from build123d import *

# Parameters (mm, degrees)
F0_R     = 9
F0_R_2   = 4
F1_DEPTH = 1.5
F2_DEPTH = 4
F3_R     = 2.35
F4_DEPTH = 2.5


# Not quite as in the source:
# - a feature names something its author has since deleted; it is built from what else it names


with BuildPart() as f1:
    # F0 (on Top) → F1 (new body)
    with BuildSketch(Plane.XY):
        Circle(F0_R)
        Circle(F0_R_2, mode=Mode.SUBTRACT)
        Circle(F0_R_2)
    extrude(amount=-F1_DEPTH)

    # F0 (on Top) → F2 (join)
    with BuildSketch(Plane.XY):
        Circle(F0_R_2)
    extrude(amount=F2_DEPTH)

    # F3 (on face) → F4 (join)
    with BuildSketch(Plane.XY.offset(4)):
        Circle(F3_R)
    extrude(amount=F4_DEPTH)


solid = f1.part
Read the model definition and answer for the solid it produces. Units are mm, in the model's axes. A direction names the side the tool comes from. Give positions to 0.01 mm unless a question says otherwise; leave off trailing zeros. Write each loop counter-clockwise with the first axis right and the second up, starting at its lowest first coordinate (ties: lowest second). Pieces come first, ordered by that corner, then holes. Notation, with made-up numbers: (-6.75, 66.25) - (49.25, 66.25) arc R13 ccw to (49.25, 85.25) - close; hole circle Ø4 at (81.25, 57). An arc over 180 degrees is marked (long way). Use CSV: the item, a comma, the result in double quotes. Start each with the question number.
(1) Consider line 1 along Z through (x, y) = (4.5, -6); line 2 along Y through (x, z) = (-0.25, 4.25); line 3 along Y through (x, z) = (0.5, 1.75). Determine where each line is inside the solid, lowest interval first.
(2) For faces 1 (the cylindrical face through (-1.172, 8.923, -0.74)), 2 (the cylindrical face through (-0.509, -2.294, 5.232)), determine the directions among +Z, -Z, +X, -X, +Y, -Y from which every point of the face is accessible in a straight line to the end or side of a thin tool.
(3) Given P1, Ø4, axis at x = 1.5, z = 2.5, coming from the +Y side; P2, Ø2, axis at x = 7, y = -4, coming from the +Z side; P3, Ø2, axis at x = -5, z = 0, coming from the +Y side, each flat-ended and moving along its own axis, determine where each tip first touches the part or whether it passes through.
(4) Find section A-A (x = 0). Give the vertices of the cut face in (y, z).
(5) Find section D-D (z = -1). Give the vertices of the cut face in (x, y).
(6) Find section C-C (z = 5.75). Give the vertices of the cut face in (x, y).
Findings below:
1,line 1,"-1.5 to 0"
1,line 2,"-2.34 to 2.34"
1,line 3,"-3.97 to 3.97"
2,face 1,"+Z, -Z"
2,face 2,"+Z"
3,P1,"y = 4"
3,P2,"z = 0"
3,P3,"y = 8.06"
4,outline,"(-9, -1.5) - (9, -1.5) - (9, 0) - (4, 0) - (4, 4) - (2.35, 4) - (2.35, 6.5) - (-2.35, 6.5) - (-2.35, 4) - (-4, 4) - (-4, 0) - (-9, 0) - close"
5,outline,"circle Ø18 at (0, 0)"
6,outline,"circle Ø4.7 at (0, 0)"
